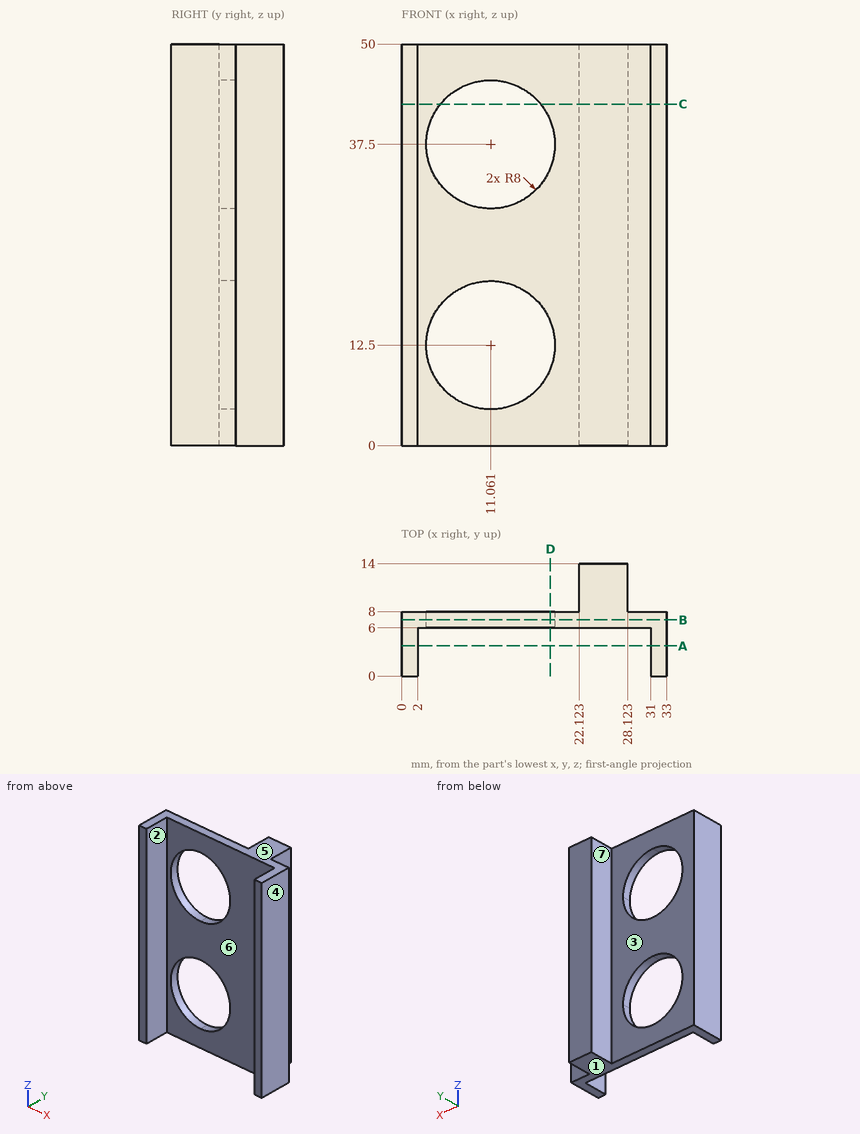
Input: dimensioned drawing with shaded views. Units: mm. Origin: part minimum x, y, z. A direction names the side the tool comes from. Coordinates: 2 decimals unless noted, no trailing zeros. Order: outer loops, then holes, each group sorted by start corner. A loop starts at its lowest first (then second) coordinate and runs counter-clockwise, first axis right, second up. Notation, with made-up numbers: (7.5, 13) -> (54.5, 13) arc R26 cw to (54.5, 42) -> close; hole circle Ø5 at (19.25, 77). An arc over 180 degrees is marked (long way). Use CSV: the item, a comma, the result in double quotes.
1) Section C-C on z = 42.5. Output: boundary loops of the cut face in (x, y).
Findings:
outline,"(0, 0) -> (2, 0) -> (2, 6) -> (4.82, 6) -> (4.82, 8) -> (0, 8) -> close; (17.31, 6) -> (31, 6) -> (31, 0) -> (33, 0) -> (33, 8) -> (28.12, 8) -> (28.12, 14) -> (22.12, 14) -> (22.12, 8) -> (17.31, 8) -> close"
2) Section D-D on x = 18.5. Output: boundary loops of the cut face in (y, z).
Findings:
outline,"(6, 0) -> (8, 0) -> (8, 9.56) -> (6, 9.56) -> close; (6, 15.44) -> (8, 15.44) -> (8, 34.56) -> (6, 34.56) -> close; (6, 40.44) -> (8, 40.44) -> (8, 50) -> (6, 50) -> close"
3) Section B-B on y = 7. Output: boundary loops of the cut face in (x, z), then the cut area to 3 significant figures.
Findings:
outline,"(0, 0) -> (33, 0) -> (33, 50) -> (0, 50) -> close; hole circle Ø16 at (11.06, 12.5); hole circle Ø16 at (11.06, 37.5)"
area,"1,250 mm^2"
4) Access query for the marked faces 1, 2 and 3. Directions: +Z, -Z, +X, -X, +Y, -Y. A direction counts if a zero-diameter tool reaches every point of the face in a straight line with its end or side. Return the directions, or none.
Findings:
face 1,"-Z, +X, -X, +Y, -Y"
face 2,"+Z, -Z, -Y"
face 3,"+Z, -Z, -X, +Y"
5) Pin query (flat end, axial travel): pin 1 Ø6.5 at (y, z) = (12, 13.5) entering from +X; pin 2 Ø2.5 at (x, z) = (29.5, 34.5) entering from +Y; pin 3 Ø3 at (y, z) = (10.5, 16) entering from -X. Return the tip coordinate at first contact, or that it passes through.
Findings:
pin 1,"stops at x = 28.12"
pin 2,"stops at y = 8"
pin 3,"stops at x = 22.12"
6) Section A-A on y = 3.75. Output: boundary loops of the cut face in (x, z), then the cut area to 3 significant figures.
Findings:
outline,"(0, 0) -> (2, 0) -> (2, 50) -> (0, 50) -> close; (31, 0) -> (33, 0) -> (33, 50) -> (31, 50) -> close"
area,"200 mm^2"
7) Mould query, pull axis X, two halves, no side actions, for the marked faces 4, 5, 6 and 7. Classes: +X half, -X half, draft (parallel to the pull), parting line (faces both ways), or undercut.
Findings:
face 4,"+X half"
face 5,"draft"
face 6,"undercut"
face 7,"-X half"
8) Line query: line 1 (X direction, y = 3, z = 39.5); line 2 (Z direction, x = 14, y = 6.5); line 3 (Y direction, x = 22, z = 35). Output: solid intervals per line, ascending.
Findings:
line 1,"x = 0 to 2, 31 to 33"
line 2,"z = 0 to 5.06, 19.94 to 30.06, 44.94 to 50"
line 3,"y = 6 to 8"
